CAD build for the part. Positions are in the model's coordinates, mm. A direction names the side the tool comes from. Give positions to 0.01 mm unless a question says otherwise; leave off trailing zeros. Loops run counter-clockwise (first coordinate to the right, second up) from the corner with the lowest first, then second, coordinate; pieces in that order, holes last.
Item 1: Saw through at D-D on y = 84.5. Give the cut face in (x, z), plus the area to 3 significant figures.
Item 2: Drop flat-ended pins along their axis: P1, Ø10, axis at x = 27.5, z = -4, coming from the +Y side; P2, Ø7.5, axis at y = 14.5, z = -15, coming from the +X side; P3, Ø8, axis at y = 78.5, z = 20, coming from the -X side. Give the stop position or say it passes through.
Item 3: Saw through at B-B on x = 0. Give the cut face in (y, z).
Item 4: Probe probe 1 along Y at (x, z) = (0, -34.5); probe 2 along X at (y, z) = (52, -26); probe 3 along Z at (x, y) = (-33.5, 39). List the from-to ranges inside material, lowest first.
Item 5: Saw through at A-A on y = 52.9. Give the cut face in (x, z).
Item 6: Mould opens along X. For faces 1 (the flat face through (-25, 12, 1)), 2 (the cylindrical face through (1.27, 90.38, -32.33)), 3 (the cylindrical face through (-3.255, 77.687, 32.675)), 4 (the cylindrical face through (-3.255, 77.687, -32.325)) say: released by +X, released by -X, zero draft, split by the parting line, or undercut.
Item 7: Saw through at C-C on x = 30.5. Give the cut face in (y, z).
Item 8: Which spindle directions (+Z, -Z, +X, -X, +Y, -Y) get a long thin tool onto all of the face, cutting with end or side? Do faces 5 (the flat face through (-1, 26, 45)), 6 (the flat face through (25, 12, 1)), 7 (the flat face through (0, 25, 0)). Say none if no direction does.
from build123d import *

# Parameters (mm, degrees)
SKETCH1_W           = 50
SKETCH1_H           = 90
BOSS_EXTRUDE1_DEPTH = 25
SKETCH2_R           = 37.5
BOSS_EXTRUDE2_DEPTH = 25
SKETCH3_R           = 25
CUT_EXTRUDE1_DEPTH  = 25
LPATTERN3_COUNT     = 2
LPATTERN3_PITCH     = 65


with BuildPart() as part:
    # Sketch1 → Boss-Extrude1 (new body)
    with BuildSketch(Plane(origin=(0, 0, 0), x_dir=(1, 0, 0), z_dir=(0, 1, 0))):
        Rectangle(SKETCH1_W, SKETCH1_H)
    extrude(amount=BOSS_EXTRUDE1_DEPTH)

    # Sketch2 → Boss-Extrude2 (add)
    with BuildSketch(Plane.XY.offset(45)):
        with Locations((0, 52.9)):
            Circle(SKETCH2_R)
    boss_extrude2 = extrude(amount=-BOSS_EXTRUDE2_DEPTH)

    # Sketch3 → Cut-Extrude1 (cut)
    with BuildSketch(Plane.XY.offset(45)):
        with Locations((0, 52.9)):
            Circle(SKETCH3_R)
    cut_extrude1 = extrude(amount=-CUT_EXTRUDE1_DEPTH, mode=Mode.SUBTRACT)

    # LPattern3: Boss-Extrude2, Cut-Extrude1 ×2
    with Locations(*[(0, 0, -i * LPATTERN3_PITCH) for i in range(1, LPATTERN3_COUNT)]):
        add(boss_extrude2)
        add(cut_extrude1, mode=Mode.SUBTRACT)


solid = part.part
Results below:
1. outline: (-20.19, -45) - (20.19, -45) - (20.19, -20) - (-20.19, -20) - close; (-20.19, 20) - (20.19, 20) - (20.19, 45) - (-20.19, 45) - close
1. area: 2,020 mm2
2. P1: stops at y = 25
2. P2: stops at x = 25
2. P3: stops at x = -30.65
3. outline: (0, -45) - (27.9, -45) - (27.9, -20) - (25, -20) - (25, 20) - (27.9, 20) - (27.9, 45) - (0, 45) - close; (77.9, -45) - (90.4, -45) - (90.4, -20) - (77.9, -20) - close; (77.9, 20) - (90.4, 20) - (90.4, 45) - (77.9, 45) - close
4. probe 1: y = 0 to 27.9, 77.9 to 90.4
4. probe 2: x = -37.49 to -24.98, 24.98 to 37.49
4. probe 3: z = -45 to -20, 20 to 45
5. outline: (-37.5, -45) - (-25, -45) - (-25, -20) - (-37.5, -20) - close; (-37.5, 20) - (-25, 20) - (-25, 45) - (-37.5, 45) - close; (25, -45) - (37.5, -45) - (37.5, -20) - (25, -20) - close; (25, 20) - (37.5, 20) - (37.5, 45) - (25, 45) - close
6. face 1: released by -X
6. face 2: split by the parting line
6. face 3: undercut
6. face 4: undercut
7. outline: (31.08, -45) - (74.72, -45) - (74.72, -20) - (31.08, -20) - close; (31.08, 20) - (74.72, 20) - (74.72, 45) - (31.08, 45) - close
8. face 5: +Z, +X, -X, +Y, -Y
8. face 6: +Z, -Z, +X, -Y
8. face 7: +X, -X, +Y
